The listing builds one solid part. Answer for the finished solid, in the listing's coordinates (mm). Face numbers are marked on the shaded views. A direction names the side the tool comes from. Round coordinates to 2 decimals unless told otherwise and drop trailing zeros. Order: outer loops, then holes, each group sorted by start corner. A loop starts at its lowest first (then second) coordinate and runs counter-clockwise, first axis right, second up. Notation, with made-up numbers: (-23.75, 9.25) - (1.25, 9.25) arc R33 cw to (1.25, 39.25) - close; hole circle Ø1 at (-25, 37.25). An arc over 180 degrees is marked (long way). Use CSV: the item, a comma, the result in double quotes. Start each with the question number.
Item 1: Find section B-B, the plane z = 15. Give the vertices of the cut face in (x, y), plus the area to 3 significant figures.
Item 2: For the marked faces 1, 2 and 3, determine the directions among +Z, -Z, +X, -X, +Y, -Y from which every point of the face is accessible in a straight line to the end or side of a thin tool.
Item 3: Find section C-C, the plane z = -5. Count the separate pieces of the cut face and the enclosed holes in it, plus the area to 3 significant figures.
Item 4: Straight lines are drawn through the part: line 1 along X through (y, z) = (5.75, -12); line 2 along Z through (x, y) = (10, 9); line 3 along Y through (x, z) = (-22, -1.5). For each, find the intervals that lie inside material, in ascending order. Write a range as [from, to].
Item 5: Flat-ended cylindrical pins translate along their axes: P1, Ø1.5, axis at x = 21, z = -13, coming from the +Y side; P2, Ø5, axis at x = 10.5, z = -5.75, coming from the -Y side; P3, Ø1.6, axis at y = -1, z = -14, coming from the +X side; P4, Ø10, axis at x = -10, y = 14, coming from the -Z side. Find the tip coordinate at first contact, or state that the pin passes through.
Item 6: Find section A-A, the plane y = 0.75. Give the vertices of the cut face in (x, z).
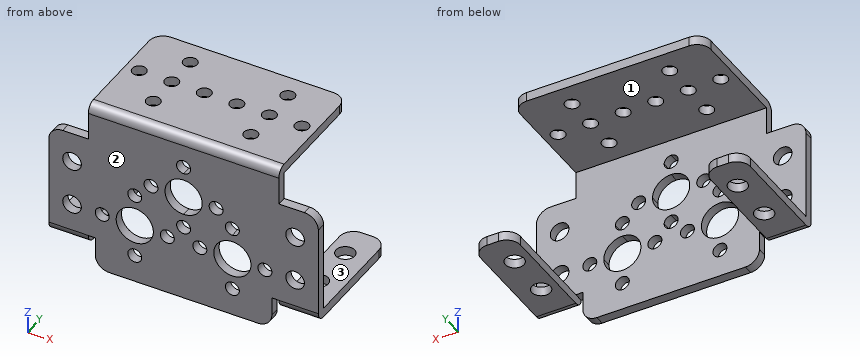
```python
from build123d import *

# Parameters (mm, degrees)
SKETCH_2_R          = 2
SKETCH_2_R_2        = 1.5
SKETCH_2_R_3        = 4
SKETCH_2_W          = 8.5
SKETCH_2_H          = 2
EXTRUDE_1_DEPTH     = 2
SKETCH_1_W          = 8.5
SKETCH_1_H          = 2
EXTRUDE_2_DEPTH     = 24
SKETCH_3_R          = 2
CUT_EXTRUDE_1_DEPTH = 12
FILLET_1_R          = 3
SKETCH_4_R          = 1.5
CUT_EXTRUDE_2_DEPTH = 12
SKETCH_5_W          = 8.5
SKETCH_5_H          = 26
CUT_EXTRUDE_3_DEPTH = 8
FILLET_2_R          = 3
FILLET_3_R          = 2


with BuildPart() as part:
    # Sketch 2 → Extrude 1 (new body)
    # profile 1 of 4: a face of its own
    with BuildSketch(Plane(origin=(0, 0, 0), x_dir=(1, 0, 0), z_dir=(0, 1, 0))):
        Polygon((-29, -16.75), (-29, -18.75), (29, -18.75), (29, -16.75), (24, -16.75), (0, -16.75), align=None)
    # profile 2 of 4: a face of its own
    with BuildSketch(Plane(origin=(0, 0, 0), x_dir=(1, 0, 0), z_dir=(0, 1, 0))):
        Polygon((-29, 11.75), (-29, -16.75), (0, -16.75), (24, -16.75), (29, -16.75), (29, 11.75), (20.5, 11.75), (19, 11.75), (19, 18.75), (-19, 18.75), (-19, 11.75), (-20.5, 11.75), align=None)
        with BuildLine():
            ThreePointArc((1.5, -11.75), (1.060660172, -12.810660172), (0, -13.25))
            ThreePointArc((0, -13.25), (-1.5, -11.75), (0, -10.25))
            ThreePointArc((0, -10.25), (1.060660172, -10.689339828), (1.5, -11.75))
        make_face(mode=Mode.SUBTRACT)
        with Locations(Location((-24, -4.25, 0), (0, 0, 270))):
            Circle(SKETCH_2_R, mode=Mode.SUBTRACT)
        with Locations(Location((-7, -4.75, 0), (0, 0, 270))):
            Circle(SKETCH_2_R_2, mode=Mode.SUBTRACT)
        with BuildLine():
            ThreePointArc((4, -4.75), (2.828427125, -7.578427125), (0, -8.75))
            ThreePointArc((0, -8.75), (-4, -4.75), (0, -0.75))
            ThreePointArc((0, -0.75), (2.828427125, -1.921572875), (4, -4.75))
        make_face(mode=Mode.SUBTRACT)
        with Locations(Location((-10.5, -1.25, 0), (0, 0, 270))):
            Circle(SKETCH_2_R_2, mode=Mode.SUBTRACT)
        with Locations(Location((7, -4.75, 0), (0, 0, 270))):
            Circle(SKETCH_2_R_2, mode=Mode.SUBTRACT)
        with BuildLine():
            ThreePointArc((12, -1.25), (9.439339828, -2.310660172), (10.5, 0.25))
            ThreePointArc((10.5, 0.25), (11.560660172, -0.189339828), (12, -1.25))
        make_face(mode=Mode.SUBTRACT)
        with Locations(Location((24, -4.25, 0), (0, 0, 270))):
            Circle(SKETCH_2_R, mode=Mode.SUBTRACT)
        with Locations(Location((-24, 5.75, 0), (0, 0, 270))):
            Circle(SKETCH_2_R, mode=Mode.SUBTRACT)
        with Locations(Location((-17.5, 5.75, 0), (0, 0, 270))):
            Circle(SKETCH_2_R_2, mode=Mode.SUBTRACT)
        with BuildLine():
            ThreePointArc((1.5, 2.25), (1.060660172, 1.189339828), (0, 0.75))
            ThreePointArc((0, 0.75), (-1.060660172, 3.310660172), (1.5, 2.25))
        make_face(mode=Mode.SUBTRACT)
        with Locations(Location((-10.5, 5.75, 0), (0, 0, 270))):
            Circle(SKETCH_2_R_3, mode=Mode.SUBTRACT)
        with Locations(Location((-3.5, 5.75, 0), (0, 0, 270))):
            Circle(SKETCH_2_R_2, mode=Mode.SUBTRACT)
        with Locations(Location((-10.5, 12.75, 0), (0, 0, 270))):
            Circle(SKETCH_2_R_2, mode=Mode.SUBTRACT)
        with Locations(Location((3.5, 5.75, 0), (0, 0, 270))):
            Circle(SKETCH_2_R_2, mode=Mode.SUBTRACT)
        with BuildLine():
            ThreePointArc((14.5, 5.75), (13.328427125, 2.921572875), (10.5, 1.75))
            ThreePointArc((10.5, 1.75), (7.671572875, 8.578427125), (14.5, 5.75))
        make_face(mode=Mode.SUBTRACT)
        with Locations(Location((17.5, 5.75, 0), (0, 0, 270))):
            Circle(SKETCH_2_R_2, mode=Mode.SUBTRACT)
        with Locations(Location((24, 5.75, 0), (0, 0, 270))):
            Circle(SKETCH_2_R, mode=Mode.SUBTRACT)
        with Locations(Location((10.5, 12.75, 0), (0, 0, 270))):
            Circle(SKETCH_2_R_2, mode=Mode.SUBTRACT)
    # profile 3 of 4: a face of its own
    with BuildSketch(Plane(origin=(0, 0, 0), x_dir=(1, 0, 0), z_dir=(0, 1, 0))):
        with Locations((-24.75, 12.75)):
            Rectangle(SKETCH_2_W, SKETCH_2_H)
    # profile 4 of 4: a face of its own
    with BuildSketch(Plane(origin=(0, 0, 0), x_dir=(1, 0, 0), z_dir=(0, 1, 0))):
        with Locations((24.75, 12.75)):
            Rectangle(SKETCH_2_W, SKETCH_2_H)
    extrude(amount=-EXTRUDE_1_DEPTH)

    # Sketch 1 → Extrude 2 (add)
    with BuildSketch(Plane(origin=(0, 0, 0), x_dir=(1, 0, 0), z_dir=(0, 1, 0))):
        with Locations((-24.75, 12.75)):
            Rectangle(SKETCH_1_W, SKETCH_1_H)
        with Locations((24.75, 12.75)):
            Rectangle(SKETCH_1_W, SKETCH_1_H)
        Polygon((-29, -16.75), (-29, -18.75), (29, -18.75), (29, -16.75), (24, -16.75), (0, -16.75), align=None)
    extrude(amount=EXTRUDE_2_DEPTH)

    # Sketch 3 → Cut-Extrude 1 (cut)
    with BuildSketch(Plane(origin=(0, 0, -13.75), x_dir=(-1, 0, 0), z_dir=(0, 0, -1))):
        with Locations((-24, 17)):
            Circle(SKETCH_3_R)
        with Locations((24, 17)):
            Circle(SKETCH_3_R)
        with Locations((24, 7)):
            Circle(SKETCH_3_R)
        with Locations((-24, 7)):
            Circle(SKETCH_3_R)
    extrude(amount=-CUT_EXTRUDE_1_DEPTH, mode=Mode.SUBTRACT)

    # Fillet 1
    fillet_1_edges = [part.edges().sort_by_distance(p)[0] for p in [
        (20.5, 24, -12.75),
        (29, 24, -12.75),
        (-29, 24, -12.75),
        (-20.5, 24, -12.75),
    ]]
    fillet(fillet_1_edges, radius=FILLET_1_R)

    # Sketch 4 → Cut-Extrude 2 (cut)
    with BuildSketch(Plane.XY.offset(18.75)):
        with Locations((10.5, 12)):
            Circle(SKETCH_4_R)
        with Locations((-10.5, 12)):
            Circle(SKETCH_4_R)
        with Locations((-17.5, 12)):
            Circle(SKETCH_4_R)
        with Locations(Location((-10.5, 19, 0), (0, 0, 180))):
            Circle(SKETCH_4_R)
        with Locations((-3.5, 12)):
            Circle(SKETCH_4_R)
        with Locations((-10.5, 5)):
            Circle(SKETCH_4_R)
        with Locations((17.5, 12)):
            Circle(SKETCH_4_R)
        with Locations((10.5, 5)):
            Circle(SKETCH_4_R)
        with Locations((3.5, 12)):
            Circle(SKETCH_4_R)
        with Locations((10.5, 19)):
            Circle(SKETCH_4_R)
    extrude(amount=-CUT_EXTRUDE_2_DEPTH, mode=Mode.SUBTRACT)

    # Sketch 5 → Cut-Extrude 3 (cut)
    with BuildSketch(Plane.XY.offset(18.75)):
        with Locations((-24.75, 11)):
            Rectangle(SKETCH_5_W, SKETCH_5_H)
        with Locations((24.75, 11)):
            Rectangle(SKETCH_5_W, SKETCH_5_H)
    extrude(amount=-CUT_EXTRUDE_3_DEPTH, mode=Mode.SUBTRACT)

    # Fillet 2
    fillet_2_edges = [part.edges().sort_by_distance(p)[0] for p in [
        (20.5, 24, 17.75),
        (-20.5, 24, 17.75),
        (-29, -1, 10.75),
        (29, -1, 10.75),
        (-19, -1, -18.75),
        (19, -1, -18.75),
    ]]
    fillet(fillet_2_edges, radius=FILLET_2_R)

    # Fillet 3
    fillet_3_edges = [part.edges().sort_by_distance(p)[0] for p in [
        (-24.75, -2, -13.75),
        (0, -2, 18.75),
        (24.75, -2, -13.75),
    ]]
    fillet(fillet_3_edges, radius=FILLET_3_R)


solid = part.part
```
Worked out:
1,outline,"(-20.5, -2) - (20.5, -2) - (20.5, 0) - (-20.5, 0) - close"
1,area,"82.0 mm²"
2,face 1,"-Z, +X, -X, +Y"
2,face 2,"+Z, -Z, +X, -X, -Y"
2,face 3,"+Z, +X, -X, +Y"
3,separate pieces,"9"
3,enclosed holes,"0"
3,area,"49.0 mm²"
4,line 1,"x = [-29, -25.56], [-22.44, -20.5], [20.5, 22.44], [25.56, 29]"
4,line 2,"z = [16.75, 18.75]"
4,line 3,"y = [-2, 0]"
5,P1,"stops at y = 23.44"
5,P2,"passes through"
5,P3,"stops at x = 29"
5,P4,"stops at z = 16.75"
6,outline,"(-29, -13.75) - (-20.5, -13.75) - (-20.5, -11.75) - (-29, -11.75) - close; (-20.5, 16.75) - (20.5, 16.75) - (20.5, 18.75) - (-20.5, 18.75) - close; (20.5, -13.75) - (29, -13.75) - (29, -11.75) - (20.5, -11.75) - close"
